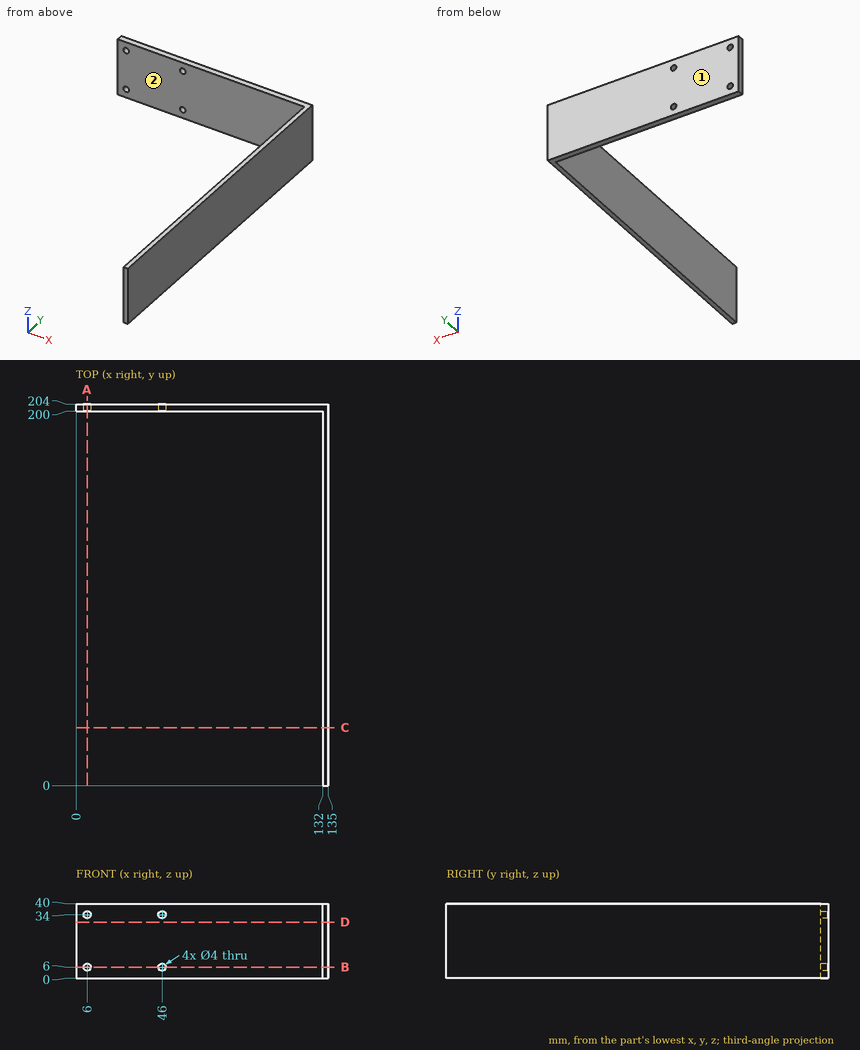
Geometry check sheet. Reference: drawing and pictorial views, mm from the part's lowest x, y, z. A direction names the side the tool comes from. Coordinates: 2 decimals unless noted, no trailing zeros. Order: outer loops, then holes, each group sorted by start corner. A loop starts at its lowest first (then second) coordinate and runs counter-clockwise, first axis right, second up. Notation, with made-up numbers: (3, -26.5) -> (19, -26.5) arc R25 cw to (19, 1.5) -> close; hole circle Ø8 at (73, -28). An arc over 180 degrees is marked (long way). Use CSV: the item, a comma, the result in double quotes. Start each with the question number.
Q1. Depth check by flat-ended pin: P1, Ø2.5, axis at x = 46, z = 34, coming from the -Y side; P2, Ø1.5, axis at x = 113.5, z = 15.5, coming from the -Y side. Enter the tip coordinate at first touch or a pass-through.
Q2. Section check A-A, the plane x = 6. Record the cut outline in (y, z), and give its area (3 significant figures).
Q3. Thickness scan on line 1 along X through (y, z) = (203.2, 6); line 2 along Y through (x, z) = (48.5, 37); line 3 along X through (y, z) = (152, 38). Record the ranges inside material, lowest first.
Q4. Tool access check on the marked faces 1 and 2. Record the directions out of +Z, -Z, +X, -X, +Y, -Y that give a thin tool (end or side, any length) a straight path to the whole face; none if there is none.
Q5. Section check D-D, the plane z = 30. Record the cut outline in (x, y), and give its area (3 significant figures).
Q6. Section check C-C, the plane y = 31. Record the cut outline in (x, z).
Q7. Section check B-B, the plane z = 6. Record the cut outline in (x, y), and give its area (3 significant figures).
Returned:
1,P1,"passes through"
1,P2,"stops at y = 200"
2,outline,"(200, 0) -> (204, 0) -> (204, 4) -> (200, 4) -> close; (200, 8) -> (204, 8) -> (204, 32) -> (200, 32) -> close; (200, 36) -> (204, 36) -> (204, 40) -> (200, 40) -> close"
2,area,"128 mm^2"
3,line 1,"x = 0 to 4, 8 to 44, 48 to 135"
3,line 2,"y = 200 to 204"
3,line 3,"x = 132 to 135"
4,face 1,"+Z, -Z, +X, -X, +Y"
4,face 2,"+Z, -Z, -X, -Y"
5,outline,"(0, 200) -> (132, 200) -> (132, 0) -> (135, 0) -> (135, 204) -> (0, 204) -> close"
5,area,"1,140 mm^2"
6,outline,"(132, 0) -> (135, 0) -> (135, 40) -> (132, 40) -> close"
7,outline,"(0, 200) -> (4, 200) -> (4, 204) -> (0, 204) -> close; (8, 200) -> (44, 200) -> (44, 204) -> (8, 204) -> close; (48, 200) -> (132, 200) -> (132, 0) -> (135, 0) -> (135, 204) -> (48, 204) -> close"
7,area,"1,110 mm^2"
